Design review of the part built by this model. Coordinates are the model's own, in mm. Face numbers are marked on the shaded views. A direction names the side the tool comes from. Round coordinates to 2 decimals unless told otherwise and drop trailing zeros. Order: outer loops, then holes, each group sorted by start corner. A loop starts at its lowest first (then second) coordinate and runs counter-clockwise, first axis right, second up. Notation, with made-up numbers: M 79.25,53 L 86.25,53 A22 cw 86.25,77 Z; hole C 26.25,26 d2. An arc over 180 degrees is marked long. Use a Markdown table: item, result. Add a question column.
(1) To check wall thickness, follow probe 1 along Y at (x, z) = (27, 7.5); probe 2 along X at (y, z) = (23, 7.5); probe 3 along X at (y, z) = (38.5, 6.5). State the ranges of each line that lie inside material, in increasing order. Write a range as from..to.
(2) Take a section at B-B (z = 2.75). Write out the cut boundary in (x, y), then the cut area to 3 significant figures.
(3) Machinability: for the marked faces 4, 5, 6 and 7, which of the approach directions +Z, -Z, +X, -X, +Y, -Y give a long, thin tool a straight path to every point of the face, cutting with its end or side? Answer none if there is none.
(4) For pin 1 (4 mm diameter, centred on x = -16, y = -4, fed in from -Z); pin 2 (2.5 mm diameter, centred on y = 40.5, z = 3.5, fed in from +X); pin 3 (2.5 mm diameter, centred on x = -23, z = 4.5, fed in from +Y), all flat-tipped, find the tip position at first contact; note any pin that passes through.
(5) The part is to be moulded in two halves that separate along X. For the marked faces 1, 2 and 3, say which applies: released by +X, released by -X, zero draft, split by the parting line, or undercut.
(6) Take a section at A-A (x = 20.5). Write out the cut boundary in (y, z), then the cut area to 3 significant figures.
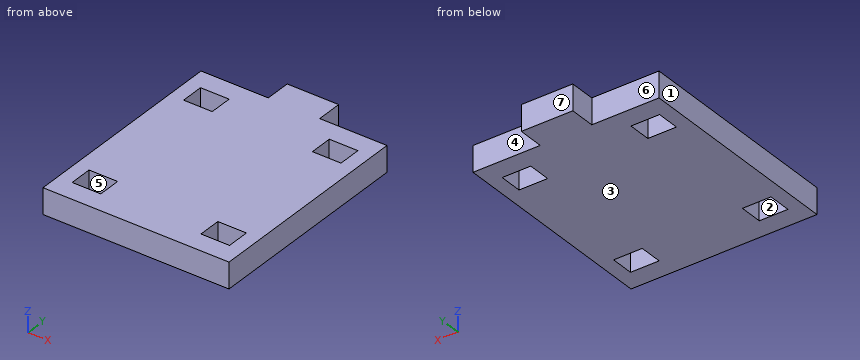
```python
from build123d import *

# Parameters (mm, degrees)
F0_W     = 65
F0_H     = 75
F1_DEPTH = 9
F3_DEPTH = 9
F4_W     = 10
F4_H     = 8
F5_DEPTH = 9.001


with BuildPart() as f1:
    # F0 (on Top) → F1 (new body)
    with BuildSketch(Plane.XY):
        Rectangle(F0_W, F0_H)
    extrude(amount=F1_DEPTH)

    # F2 (on face) → F3 (join, through all)
    with BuildSketch(Plane.XY.offset(9)):
        Polygon((9, 46.5), (0, 46.5), (-9, 46.5), (-9, 37.5), (0, 37.5), (9, 37.5), align=None)
    extrude(amount=-F3_DEPTH)

    # F4 (on face) → F5 (cut, through all)
    with BuildSketch(Plane.XY.offset(9)):
        with Locations((-22.5, 26.4595)):
            Rectangle(F4_W, F4_H)
        with Locations((22.5, 26.4595)):
            Rectangle(F4_W, F4_H)
        with Locations((22.5, -26.4595)):
            Rectangle(F4_W, F4_H)
        with Locations((-22.5, -26.4595)):
            Rectangle(F4_W, F4_H)
    extrude(amount=-F5_DEPTH, mode=Mode.SUBTRACT)


solid = f1.part
```
Verdict:
| question | item | result |
|---|---|---|
| 1 | probe 1 | y = -37.5..-30.46, -22.46..22.46, 30.46..37.5 |
| 1 | probe 2 | x = -32.5..-27.5, -17.5..17.5, 27.5..32.5 |
| 1 | probe 3 | x = -9..9 |
| 2 | outline | M -32.5,-37.5 L 32.5,-37.5 L 32.5,37.5 L 9,37.5 L 9,46.5 L -9,46.5 L -9,37.5 L -32.5,37.5 Z; hole M -27.5,-30.46 L -17.5,-30.46 L -17.5,-22.46 L -27.5,-22.46 Z; hole M -27.5,22.46 L -17.5,22.46 L -17.5,30.46 L -27.5,30.46 Z; hole M 17.5,-30.46 L 27.5,-30.46 L 27.5,-22.46 L 17.5,-22.46 Z; hole M 17.5,22.46 L 27.5,22.46 L 27.5,30.46 L 17.5,30.46 Z |
| 2 | area | 4,720 mm^2 |
| 3 | face 4 | +Z, -Z, +X, +Y |
| 3 | face 5 | +Z, -Z |
| 3 | face 6 | +Z, -Z, -X, +Y |
| 3 | face 7 | +Z, -Z, +X, -X, +Y |
| 4 | pin 1 | stops at z = 0 |
| 4 | pin 2 | stops at x = 9 |
| 4 | pin 3 | stops at y = 37.5 |
| 5 | face 1 | released by -X |
| 5 | face 2 | undercut |
| 5 | face 3 | zero draft |
| 6 | outline | M -37.5,0 L -30.46,0 L -30.46,9 L -37.5,9 Z; M -22.46,0 L 22.46,0 L 22.46,9 L -22.46,9 Z; M 30.46,0 L 37.5,0 L 37.5,9 L 30.46,9 Z |
| 6 | area | 531 mm^2 |
